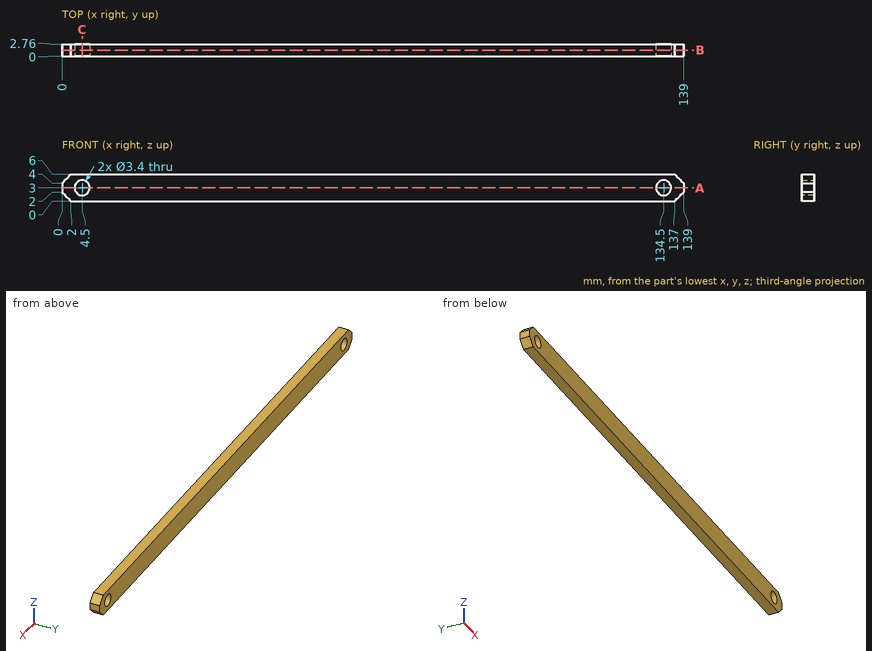
Here's the drawing with two shaded views (mm, measured from the low corner). I have some questions. Give positions to 0.01 mm unless a question says otherwise; leave off trailing zeros. Order: outer loops, then holes, each group sorted by start corner. A loop starts at its lowest first (then second) coordinate and runs counter-clockwise, first axis right, second up.
Q1. Suppose I cut it at A-A, the plane z = 3. Write out the boundary of the cut face in (x, y), and give its area (3 significant figures).
Q2. Suppose I cut it at C-C, the plane x = 4.5. Write out the boundary of the cut face in (y, z), and give its area (3 significant figures).
Q3. Suppose I cut it at B-B, the plane y = 1.4. Write out the boundary of the cut face in (x, z).
Q4. If I drill on line 1 along X through (y, z) = (1.55, 3); line 2 along X through (y, z) = (2.3, 2.25); line 3 along Z through (x, y) = (134.5, 0.65), over which ranges is the centre line in solid material (lowest first)?
Solution:
1. outline: (0, 0) - (2.8, 0) - (2.8, 2.76) - (0, 2.76) - close; (6.2, 0) - (132.8, 0) - (132.8, 2.76) - (6.2, 2.76) - close; (136.2, 0) - (139, 0) - (139, 2.76) - (136.2, 2.76) - close
1. area: 365 mm2
2. outline: (0, 0) - (2.76, 0) - (2.76, 1.3) - (0, 1.3) - close; (0, 4.7) - (2.76, 4.7) - (2.76, 6) - (0, 6) - close
2. area: 7.18 mm2
3. outline: (0, 2) - (2, 0) - (137, 0) - (139, 2) - (139, 4) - (137, 6) - (2, 6) - (0, 4) - close; hole circle Ø3.4 at (4.5, 3); hole circle Ø3.4 at (134.5, 3)
4. line 1: x = 0 to 2.8, 6.2 to 132.8, 136.2 to 139
4. line 2: x = 0 to 2.97, 6.03 to 132.97, 136.03 to 139
4. line 3: z = 0 to 1.3, 4.7 to 6
